```python
from build123d import *

# Parameters (mm, degrees)
BOSS_SWITCH_BODY_DEPTH        = 3
SKETCH1_W                     = 4
SKETCH1_H                     = 3.687347025
SKETCH1_H_2                   = 4.149321045
BOSS_FLANGE_WIDTH_DEPTH       = 5
BOSS_FLANGE_HEIGHT_REACH      = 35.973
SKETCH2_W                     = 4
SKETCH2_H                     = 4.149321045
SKETCH2_W_2                   = 8
SKETCH2_H_2                   = 2.53802598
SKETCH17_W                    = 14.933333866
SKETCH17_H                    = 4
BOSS_FLANGE_SUPPORT_DEPTH     = 10.812652975
CUT_WALL_GAP_DEPTH            = 1
SKETCH26_W                    = 10.933333866
SKETCH26_H                    = 6
CUT_CAM_SLOPE_CLEARANCE_DEPTH = 31.059873248
TAP_DRILL_FOR_M2X0_4_TAP1_D   = 1.6
M2_CLEARANCE_HOLE2_D          = 2.4
M2_CLEARANCE_HOLE2_DEPTH      = 6.5
CHAMFER_FLANGE_SUPPORT_3_SIZE = 1
SKETCH25_W                    = 5.60571229
SKETCH25_H                    = 17.5
CUT_BASE_REMOVAL_DEPTH        = 3
CHAMFER8_SIZE                 = 2.5
FILLET1_R                     = 1
FILLET2_R                     = 0.5


with BuildPart() as part:
    # Sketch-SwitchBossUp → Boss-Switch Body (new body)
    with BuildSketch(Plane.XY):
        with BuildLine():
            Line((-0.897289862, 21.27382814), (-0.700379438, 19.929528492))
            ThreePointArc((-0.700379438, 19.929528492), (-1.357570909, 19.537245674), (-1.544889614, 18.795155289))
            Line((-1.544889614, 18.795155289), (-1.110095072, 15.826830221))
            ThreePointArc((-1.110095072, 15.826830221), (-0.717812255, 15.169638751), (0.02427813, 14.982320046))
            Line((0.02427813, 14.982320046), (0.840131285, 9.412522958))
            Line((0.840131285, 9.412522958), (1.945259485, 8.880589721))
            Line((1.945259485, 8.880589721), (2.553471215, 8.587838134))
            Line((2.553471215, 8.587838134), (2.104108424, 7.654255765))
            ThreePointArc((2.104108424, 7.654255765), (2.079372028, 7.545829251), (2.104108424, 7.437402737))
            Line((2.104108424, 7.437402737), (2.553471215, 6.503820369))
            Line((2.553471215, 6.503820369), (1.945259485, 6.211068782))
            Line((1.945259485, 6.211068782), (3.246377649, 3.507905538))
            Line((3.246377649, 3.507905538), (3.854589379, 3.800657125))
            Line((3.854589379, 3.800657125), (4.722001489, 1.998548296))
            Line((4.722001489, 1.998548296), (3.820947074, 1.564842241))
            Line((3.820947074, 1.564842241), (3.820947074, -0.973183739))
            Line((3.820947074, -0.973183739), (5.277352178, -0.973183739))
            Line((5.277352178, -0.973183739), (13.426659364, -0.973183739))
            Line((13.426659364, -0.973183739), (13.426659364, 16.526816261))
            Line((13.426659364, 16.526816261), (7.114618425, 16.526816261))
            Line((7.114618425, 16.526816261), (3.820947074, 16.526816261))
            Line((3.820947074, 16.526816261), (3.820947074, 13.526816261))
            Line((3.820947074, 13.526816261), (4.722001489, 13.093110206))
            Line((4.722001489, 13.093110206), (3.854589379, 11.291001377))
            Line((3.854589379, 11.291001377), (2.490115752, 11.94776579))
            Line((2.490115752, 11.94776579), (1.110059725, 21.369353491))
            ThreePointArc((1.110059725, 21.369353491), (2.982945849, 23.574065074), (2.208754741, 26.361372687))
            ThreePointArc((2.208754741, 26.361372687), (1.148478545, 26.389910192), (1.119941041, 25.329633996))
            ThreePointArc((1.119941041, 25.329633996), (0.033089246, 22.651561394), (-1.270789677, 25.230944933))
            ThreePointArc((-1.270789677, 25.230944933), (-1.386617314, 26.285261754), (-2.440934135, 26.169434117))
            ThreePointArc((-2.440934135, 26.169434117), (-2.976976555, 23.309245483), (-0.897289862, 21.27382814))
        make_face()
        with BuildLine():
            Line((6.208741273, 2.714163286), (10.695012416, 2.714163286))
            Line((10.695012416, 2.714163286), (10.695012416, 12.377495216))
            Line((10.695012416, 12.377495216), (6.208741273, 12.377495216))
            Line((6.208741273, 12.377495216), (5.307686858, 12.811201271))
            Line((5.307686858, 12.811201271), (4.440274749, 11.009092442))
            Line((4.440274749, 11.009092442), (5.048486478, 10.716340855))
            Line((5.048486478, 10.716340855), (3.747368314, 8.013177611))
            Line((3.747368314, 8.013177611), (3.139156584, 8.305929198))
            Line((3.139156584, 8.305929198), (2.825485502, 7.654255765))
            ThreePointArc((2.825485502, 7.654255765), (2.800749105, 7.545829251), (2.825485502, 7.437402737))
            Line((2.825485502, 7.437402737), (3.139156584, 6.785729304))
            Line((3.139156584, 6.785729304), (3.747368314, 7.078480891))
            Line((3.747368314, 7.078480891), (5.048486478, 4.375317648))
            Line((5.048486478, 4.375317648), (4.440274749, 4.082566061))
            Line((4.440274749, 4.082566061), (5.307686858, 2.280457231))
            Line((5.307686858, 2.280457231), (6.208741273, 2.714163286))
        make_face(mode=Mode.SUBTRACT)
    extrude(amount=BOSS_SWITCH_BODY_DEPTH)

    # Sketch1 → Boss-Flange Width (add)
    with BuildSketch(Plane(origin=(0, 0, 0), x_dir=(-1, 0, 0), z_dir=(0, 0, -1))):
        with Locations((-5.820947074, 0.870489774)):
            Rectangle(SKETCH1_W, SKETCH1_H)
        with Locations((-5.820947074, 14.452155739)):
            Rectangle(SKETCH1_W, SKETCH1_H_2)
    extrude(amount=BOSS_FLANGE_WIDTH_DEPTH)

    # Sketch2 → Boss-Flange Height (add, up to next)
    with BuildSketch(Plane(origin=(-7.112386792, 0, 0), x_dir=(0, 0, -1), z_dir=(1, 0, 0)), mode=Mode.PRIVATE) as boss_flange_height_sk1:
        with Locations((3, 14.452155739)):
            Rectangle(SKETCH2_W, SKETCH2_H)
    boss_flange_height_tool1 = extrude(boss_flange_height_sk1.sketch, amount=BOSS_FLANGE_HEIGHT_REACH, mode=Mode.PRIVATE) - part.part
    # Sketch2 → Boss-Flange Height (add, up to next)
    with BuildSketch(Plane(origin=(-7.112386792, 0, 0), x_dir=(0, 0, -1), z_dir=(1, 0, 0)), mode=Mode.PRIVATE) as boss_flange_height_sk2:
        with Locations((1, 0.295829251)):
            Rectangle(SKETCH2_W_2, SKETCH2_H_2)
    boss_flange_height_tool2 = extrude(boss_flange_height_sk2.sketch, amount=BOSS_FLANGE_HEIGHT_REACH, mode=Mode.PRIVATE) - part.part
    add(boss_flange_height_tool1.solids().sort_by_distance((-7.112387, 14.452156, -3))[0])
    add(boss_flange_height_tool2.solids().sort_by_distance((-7.112387, 0.295829, -1))[0])

    # Sketch17 → Boss-Flange Support (add)
    with BuildSketch(Plane.XZ.offset(-1.564842241)):
        with Locations((0.354280141, -3)):
            Rectangle(SKETCH17_W, SKETCH17_H)
    extrude(amount=-BOSS_FLANGE_SUPPORT_DEPTH)

    # Sketch27 → Cut-Wall Gap (cut)
    with BuildSketch(Plane.XY):
        Polygon((3.820947074, 13.526816261), (6.208741273, 12.377495216), (3.820947074, 12.377495216), align=None)
        Polygon((6.208741273, 2.714163286), (3.820947074, 2.714163286), (3.820947074, 1.564842241), align=None)
    extrude(amount=-CUT_WALL_GAP_DEPTH, mode=Mode.SUBTRACT)

    # Sketch26 → Cut-Cam Slope Clearance (cut, through all)
    with BuildSketch(Plane.XY.offset(-1)):
        with Locations((-1.645719859, 13.526816261)):
            Rectangle(SKETCH26_W, SKETCH26_H)
    extrude(amount=-CUT_CAM_SLOPE_CLEARANCE_DEPTH, mode=Mode.SUBTRACT)

    # Tap Drill for M2x0.4 Tap1 (through all)
    with Locations(Plane(origin=(0, -0.973183739, 0), x_dir=(-1, 0, 0), z_dir=(0, -1, 0))):
        with Locations((4.112386792, 3), (-5.320947074, 3)):
            Hole(TAP_DRILL_FOR_M2X0_4_TAP1_D / 2)

    # M2 Clearance Hole2
    with Locations(Plane.XZ.offset(0.973183739)):
        with Locations((-4.112386792, -3), (5.320947074, -3)):
            Hole(M2_CLEARANCE_HOLE2_D / 2, depth=M2_CLEARANCE_HOLE2_DEPTH)

    # Chamfer-Flange Support 3
    chamfer_flange_support_3_edges = [part.edges().sort_by_distance(p)[0] for p in [
        (-1.645719859, 1.564842241, -1),
    ]]
    chamfer(chamfer_flange_support_3_edges, length=CHAMFER_FLANGE_SUPPORT_3_SIZE)

    # Sketch25 → Cut-Base Removal (cut)
    with BuildSketch(Plane.XY.offset(3)):
        with Locations((10.623803219, 7.776816261)):
            Rectangle(SKETCH25_W, SKETCH25_H)
    extrude(amount=-CUT_BASE_REMOVAL_DEPTH, mode=Mode.SUBTRACT)

    # Chamfer8
    # the kernel refuses this chamfer: 2.5 mm, written as the material it takes off along each edge
    with BuildSketch(Plane(origin=(14.250154544, 16.526816261, -5), x_dir=(0, 0.027495876610586317, 0.9996219169112968), z_dir=(-1, 0, 0))) as chamfer8_piece_1:
        Polygon((CHAMFER8_SIZE * 0.999621916911, -CHAMFER8_SIZE * 0.0274958766106), (-CHAMFER8_SIZE * 0.0274958766106, -CHAMFER8_SIZE * 0.999621916911), (0, 0), align=None)
    extrude(amount=16.85841494, mode=Mode.SUBTRACT)

    # Fillet1
    fillet1_edges = [part.edges().sort_by_distance(p)[0] for p in [
        (0.840131285, 9.412522958, 1.5),
    ]]
    fillet(fillet1_edges, radius=FILLET1_R)

    # Fillet2
    fillet2_edges = [part.edges().sort_by_distance(p)[0] for p in [
        (1.945259485, 6.211068782, 1.5),
    ]]
    fillet(fillet2_edges, radius=FILLET2_R)


solid = part.part
```
The listing builds one solid part. Answer for the finished solid, in the listing's coordinates (mm). A direction names the side the tool comes from. Coordinates: 2 decimals unless noted, no trailing zeros. Loops run counter-clockwise (first coordinate to the right, second up) from the corner with the lowest first, then second, coordinate; pieces in that order, holes last. Notation, with made-up numbers: (-10, 36.25) -> (11, 36.25) arc R22 ccw to (11, 58.25) -> close; hole circle Ø4 at (33.25, -2.75). An arc over 180 degrees is marked (long way). Return JSON: item names as keys, results as strings. Group by question number.
(1) A cutting plane is placed at A-A on z = -3.5. Write down the section's boundary in (x, y).
(2) Given pin 1 Ø1.9 at (x, z) = (5.32, -3) entering from +Y; pin 2 Ø1.9 at (x, z) = (-4.11, -3) entering from +Y; pin 3 Ø2.5 at (x, y) = (1, 13) entering from -Z, each flat-ended and moving along its own axis, determine where each tip first touches the part or whether it passes through.
(3) Which of the six approach directions +Z, -Z, +X, -X, +Y, -Y give full straight-line access (tool end or side, diameter ignored) to faces 4 (the flat face through (4.87, 3.19, 1.48)), 5 (the flat face through (-2, 1.565, 2)), 6 (the cylindrical face through (5.48, 2.32, -1.81)), 7 (the flat face through (-2, 10.527, -3))?
(4) A cutting plane is placed at B-B on y = 17.5. Write down the section's boundary in (x, z), and give its area (3 significant figures).
(5) Find the intervals of material crossed by probe 1 along X at (y, z) = (8.8, -3); probe 2 along Y at (x, z) = (6.75, 0.5); probe 3 along X at (y, z) = (1.5, -2.25), in increasing order. Write a range as from..to.
(6) Determine the mould class of faces 1 (the flat face through (7.821, 8, -2)), 2 (the flat face through (3.182, 11.615, 1.479)), 3 (the flat face through (1, 16, 0)) for opening direction X: released by +X, released by -X, zero draft, split by the parting line, or undercut.
The answers:
{
 "1": {"outline": "(-7.11, -0.97) -> (-5.2, -0.97) -> (-5.2, 5.53) -> (-4.74, 5.53) -> (-4.74, 10.53) -> (-7.11, 10.53) -> close; (-3.49, 5.53) -> (-3.02, 5.53) -> (-3.02, -0.97) -> (4.23, -0.97) -> (4.23, 5.53) -> (4.7, 5.53) -> (4.7, 15.53) -> (3.82, 15.53) -> (3.82, 10.53) -> (-3.49, 10.53) -> close; (5.95, 5.53) -> (6.41, 5.53) -> (6.41, -0.97) -> (7.82, -0.97) -> (7.82, 15.53) -> (5.95, 15.53) -> close"},
 "2": {"pin 1": "stops at y = 16.53", "pin 2": "stops at y = 10.53", "pin 3": "stops at z = 0"},
 "3": {"face 4": "+Z", "face 5": "+Z, -X", "face 6": "-Y", "face 7": "-Z, -X, +Y"},
 "4": {"outline": "(-1.36, 0) -> (1.68, 0) -> (1.68, 3) -> (-1.36, 3) -> close", "area": "9.10 mm^2"},
 "5": {"probe 1": "x = -7.11..-4.91, -3.31..4.52, 6.12..7.82", "probe 2": "y = -0.97..2.71, 12.38..16.53", "probe 3": "x = -7.11..-5.05, -3.18..4.38, 6.26..7.82"},
 "6": {"face 1": "released by +X", "face 2": "undercut", "face 3": "zero draft"}
}
